Part model, mm, in its own coordinate system. Give positions to 0.01 mm unless a question says otherwise; leave off trailing zeros. Order: outer loops, then holes, each group sorted by start corner. A loop starts at its lowest first (then second) coordinate and runs counter-clockwise, first axis right, second up. Notation, with made-up numbers: (50, -36.5) -> (73, -36.5) arc R10 ccw to (73, -22.5) -> close; hole circle Ø7 at (49.5, 44). An arc over 180 degrees is marked (long way). Write item = value, one per line. Start each with the question number.
Item 1: Drill centre lines: line 1 along Y through (x, z) = (153.5, -387); line 2 along X through (y, z) = (753, 286); line 3 along Z through (x, y) = (-231.5, 44). Where is each one in solid material? Low to high.
Item 2: Flat gauge pins, fed straight in: P1, Ø9, axis at y = 278.5, z = -481.5, coming from the +X side; P2, Ø6, axis at x = -456, z = -478.5, coming from the -Y side; P3, Ø12, axis at y = 41, z = -262, coming from the +X side. Where does each tip first touch, or does it go through?
Item 3: Band-saw the part on D-D on x = -886.5. Write the cut outline in (y, z), plus the area to 3 significant figures.
Item 4: Band-saw the part on C-C on z = 53.5. Write the cut outline in (x, y).
Item 5: Band-saw the part on B-B on y = 676. Write the cut outline in (x, z), plus the area to 3 significant figures.
Item 6: Band-saw the part on A-A on x = 308. Write the cut outline in (y, z).
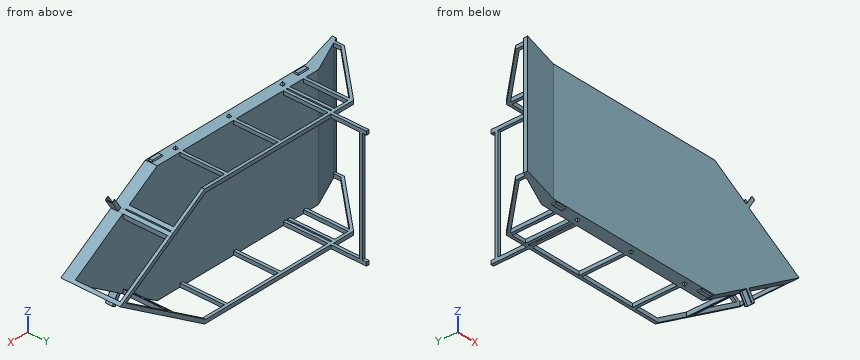
```python
from build123d import *

# Parameters (mm, degrees)
BOSS_EXTRUDE1_DEPTH      = 500
BOSS_EXTRUDE2_DEPTH      = 500
BOSS_EXTRUDE2_DEPTH_BACK = 500
CUT_EXTRUDE1_START       = -500
CUT_EXTRUDE1_OUTLINE_W   = 473.864747831
CUT_EXTRUDE1_OUTLINE_H   = 375
CUT_EXTRUDE1_OUTLINE_W_2 = 7.552750907
CUT_EXTRUDE1_OUTLINE_W_3 = 441.311996924
CUT_EXTRUDE1_OUTLINE_W_4 = 436.609859473
CUT_EXTRUDE1_OUTLINE_W_5 = 473.864747832
CUT_EXTRUDE1_OUTLINE_W_6 = 12.254888358
CUT_EXTRUDE1_OUTLINE_W_7 = 125
CUT_EXTRUDE1_DEPTH       = 1000
BOSS_EXTRUDE3_DEPTH      = 100
CUT_EXTRUDE4_DEPTH       = 470
BOSS_EXTRUDE5_DEPTH      = 500
BOSS_EXTRUDE5_DEPTH_BACK = 500
CUT_EXTRUDE7_DEPTH       = 470
SKETCH10_W               = 1000
SKETCH10_H               = 25
BOSS_EXTRUDE6_DEPTH      = 25
SKETCH11_W               = 25
SKETCH11_H               = 25
SKETCH11_W_2             = 24.921787331
BOSS_EXTRUDE7_DEPTH      = 25
BOSS_EXTRUDE7_TAPER      = 30
BOSS_EXTRUDE8_START      = 525.229495663
BOSS_EXTRUDE8_DEPTH      = 0.022340747
BOSS_EXTRUDE8_START_2    = -485
BOSS_EXTRUDE8_2_DEPTH    = 25
BOSS_EXTRUDE8_START_3    = 13.864747831
BOSS_EXTRUDE8_3_DEPTH    = 25
BOSS_EXTRUDE8_START_4    = 512.729495663
BOSS_EXTRUDE8_4_DEPTH    = 25.022340747
BOSS_EXTRUDE8_START_5    = 37
BOSS_EXTRUDE8_5_DEPTH    = 26
BOSS_EXTRUDE10_DEPTH     = 500
CUT_EXTRUDE8_DEPTH       = 440
CUT_EXTRUDE9_DEPTH       = 23
CUT_EXTRUDE10_DEPTH      = 23
SKETCH20_W               = 100
SKETCH20_H               = 40
BOSS_EXTRUDE11_DEPTH     = 10
BOSS_EXTRUDE11_TAPER     = 29
SKETCH22_W               = 100
SKETCH22_H               = 40
BOSS_EXTRUDE12_DEPTH     = 10
BOSS_EXTRUDE12_TAPER     = 29


with BuildPart() as part:
    # Sketch3 → Boss-Extrude1 (new body)
    with BuildSketch(Plane(origin=(0, 0, 0), x_dir=(1, 0, 0), z_dir=(0, 1, 0))):
        Polygon((750, -500), (1535.458991325, 0), (750, 500), (-750, 500), (-750, -500), align=None)
        Polygon((741.261584038, -470), (1479.593035884, 0), (741.261584038, 470), (-720, 470), (-720, -470), align=None, mode=Mode.SUBTRACT)
    extrude(amount=BOSS_EXTRUDE1_DEPTH)

    # Sketch4 → Boss-Extrude2 (add, two sides: drawn at the far end of the back side and taken through both)
    with BuildSketch(Plane.XY.offset(-BOSS_EXTRUDE2_DEPTH_BACK)):
        Polygon((-750, 0), (-750, 100), (-1044.23243351, -38.029978885), (-1044.23243351, 21.970021115), (-635, 466.05675301), (-635, 500), (-1066.865697626, 31.352330432), (-1066.865697626, -48.647669568), (-1096.782201963, -62.68206548), (-1096.782201963, -97.017235637), align=None)
    extrude(amount=BOSS_EXTRUDE2_DEPTH + BOSS_EXTRUDE2_DEPTH_BACK)

    # Cut-Extrude1: read off the stored shape, not the designer's step
    # Cut-Extrude1 outline → Cut-Extrude1 (cut)
    with BuildSketch(Plane.XY.offset(CUT_EXTRUDE1_START)):
        Polygon((-635, 100), (-635, 466.05675301), (-750, 341.262210872), (-750, 100), align=None)
        with Locations((774.661869579, 287.5)):
            Rectangle(CUT_EXTRUDE1_OUTLINE_W, CUT_EXTRUDE1_OUTLINE_H)
        with Locations((1040.370618948, 287.5)):
            Rectangle(CUT_EXTRUDE1_OUTLINE_W_2, CUT_EXTRUDE1_OUTLINE_H)
        with Locations((1289.802992863, 287.5)):
            Rectangle(CUT_EXTRUDE1_OUTLINE_W_3, CUT_EXTRUDE1_OUTLINE_H)
        with Locations((-204.440181906, 287.5)):
            Rectangle(CUT_EXTRUDE1_OUTLINE_W_4, CUT_EXTRUDE1_OUTLINE_H)
        with Locations((275.797121747, 287.5)):
            Rectangle(CUT_EXTRUDE1_OUTLINE_W_5, CUT_EXTRUDE1_OUTLINE_H)
        with Locations((-453.872555821, 287.5)):
            Rectangle(CUT_EXTRUDE1_OUTLINE_W_6, CUT_EXTRUDE1_OUTLINE_H)
        with Locations((-547.5, 287.5)):
            Rectangle(CUT_EXTRUDE1_OUTLINE_W_7, CUT_EXTRUDE1_OUTLINE_H)
        Polygon((-750, 375.205457862), (-635, 500), (-750, 500), align=None)
    extrude(amount=CUT_EXTRUDE1_DEPTH, mode=Mode.SUBTRACT)

    # Sketch3<6> → Boss-Extrude3 (add)
    with BuildSketch(Plane(origin=(0, 0, 0), x_dir=(1, 0, 0), z_dir=(0, 1, 0))):
        Polygon((750, -500), (1535.458991325, 0), (750, 500), (-750, 500), (-750, -500), align=None)
    extrude(amount=BOSS_EXTRUDE3_DEPTH)

    # Sketch4<6> → Cut-Extrude4 (cut, symmetric)
    with BuildSketch(Plane.XY):
        Polygon((-1066.865697626, -48.647669568), (-1044.23243351, -38.029978885), (-1044.23243351, 21.970021115), (-750, 341.262210872), (-635, 466.05675301), (-635, 500), (-750, 375.205457862), (-1066.865697626, 31.352330432), align=None)
    extrude(amount=CUT_EXTRUDE4_DEPTH, both=True, mode=Mode.SUBTRACT)

    # Sketch4<7> → Boss-Extrude5 (add, two sides: drawn at the far end of the back side and taken through both)
    with BuildSketch(Plane.XY.offset(-BOSS_EXTRUDE5_DEPTH_BACK)):
        Polygon((-447.745111642, 475), (-447.745111642, 100), (-422.745111642, 100), (-422.745111642, 475), (-422.745111642, 500), (-422.745111642, 800), (-447.745111642, 800), (-447.745111642, 500), align=None)
    extrude(amount=BOSS_EXTRUDE5_DEPTH + BOSS_EXTRUDE5_DEPTH_BACK)

    # Sketch4<8> → Cut-Extrude7 (cut, symmetric)
    with BuildSketch(Plane.XY):
        Polygon((-447.745111642, 475), (-447.745111642, 100), (-422.745111642, 100), (-422.745111642, 475), (-422.745111642, 500), (-422.745111642, 800), (-447.745111642, 800), (-447.745111642, 500), align=None)
    extrude(amount=CUT_EXTRUDE7_DEPTH, both=True, mode=Mode.SUBTRACT)

    # Sketch10 → Boss-Extrude6 (add)
    with BuildSketch(Plane.ZY.offset(447.745111642)):
        with Locations((0, 752.218873566)):
            Rectangle(SKETCH10_W, SKETCH10_H)
    extrude(amount=-BOSS_EXTRUDE6_DEPTH)

    # Sketch11 → Boss-Extrude7 (add)
    with BuildSketch(Plane.XY.offset(500)):
        with Locations((525.229495663, 50)):
            Rectangle(SKETCH11_W, SKETCH11_H)
        with Locations((26.364747831, 50)):
            Rectangle(SKETCH11_W, SKETCH11_H)
        with Locations((-472.460893666, 50)):
            Rectangle(SKETCH11_W_2, SKETCH11_H)
    extrude(amount=BOSS_EXTRUDE7_DEPTH, taper=BOSS_EXTRUDE7_TAPER)

    # Boss-Extrude8: read off the stored shape, not the designer's step
    # Boss-Extrude8 outline → Boss-Extrude8 (add)
    with BuildSketch(Plane.YZ.offset(BOSS_EXTRUDE8_START)):
        Polygon((62.5, -500), (37.5, -500), (50, -521.650635095), align=None)
    extrude(amount=BOSS_EXTRUDE8_DEPTH)

    # Boss-Extrude8 2 outline → Boss-Extrude8 2 (add)
    with BuildSketch(Plane.YZ.offset(BOSS_EXTRUDE8_START_2)):
        Polygon((62.5, -500), (37.5, -500), (50, -521.650635095), align=None)
    extrude(amount=BOSS_EXTRUDE8_2_DEPTH)

    # Boss-Extrude8 3 outline → Boss-Extrude8 3 (add)
    with BuildSketch(Plane.YZ.offset(BOSS_EXTRUDE8_START_3)):
        Polygon((62.5, -500), (37.5, -500), (50, -521.650635095), align=None)
    extrude(amount=BOSS_EXTRUDE8_3_DEPTH)

    # Boss-Extrude8 4 outline → Boss-Extrude8 4 (add)
    with BuildSketch(Plane.YZ.offset(BOSS_EXTRUDE8_START_4)):
        Polygon((62.5, -500), (37.5, -500), (50, -521.650635095), align=None)
    extrude(amount=BOSS_EXTRUDE8_4_DEPTH)

    # Boss-Extrude8 5 outline → Boss-Extrude8 5 (cut)
    with BuildSketch(Plane(origin=(0, 0, 0), x_dir=(1, 0, 0), z_dir=(0, 1, 0)).offset(BOSS_EXTRUDE8_START_5)):
        Polygon((512.729495663, 500), (525.229495663, 521.650635095), (525.240666036, 521.669982749), (524.472780219, 523), (512.729495663, 523), align=None)
        Polygon((526.008551854, 523), (525.240666036, 521.669982749), (525.25183641, 521.650635095), (537.75183641, 500), (537.75183641, 523), align=None)
        Polygon((38.864747831, 500), (38.864747831, 523), (13.864747831, 523), (13.864747831, 500), (26.364747831, 521.650635095), align=None)
        Polygon((-460, 500), (-460, 523), (-485, 523), (-485, 500), (-472.5, 521.650635095), align=None)
    extrude(amount=BOSS_EXTRUDE8_5_DEPTH, mode=Mode.SUBTRACT)

    # Sketch15 → Boss-Extrude10 (add)
    with BuildSketch(Plane(origin=(0, 500, 0), x_dir=(1, 0, 0), z_dir=(0, 1, 0))):
        Polygon((1069.146994401, -296.84044748), (1044.146994401, -312.754709253), (1097.846962052, -397.112954104), (1122.846962052, -381.198692331), align=None)
        Polygon((1044.146994401, 312.754709253), (1097.846962052, 397.112954104), (1122.846962052, 381.198692331), (1069.146994401, 296.84044748), align=None)
    extrude(amount=-BOSS_EXTRUDE10_DEPTH)

    # Sketch15<2> → Cut-Extrude8 (cut)
    with BuildSketch(Plane(origin=(0, 500, 0), x_dir=(1, 0, 0), z_dir=(0, 1, 0))):
        Polygon((1069.146994401, -296.84044748), (1044.146994401, -312.754709253), (1097.846962052, -397.112954104), (1122.846962052, -381.198692331), align=None)
        Polygon((1044.146994401, 312.754709253), (1097.846962052, 397.112954104), (1122.846962052, 381.198692331), (1069.146994401, 296.84044748), align=None)
    extrude(amount=-CUT_EXTRUDE8_DEPTH, mode=Mode.SUBTRACT)

    # Sketch17 → Cut-Extrude9 (cut)
    with BuildSketch(Plane(origin=(601.368753994, 0, -382.813590929), x_dir=(0.5369996765096833, 0, 0.8435824485066624), z_dir=(-0.8435824485066624, 0, 0.5369996765096833))):
        Polygon((824.540981636, 5), (919.540981636, 5), (968.552500425, 5), (968.552500425, 55), (924.540981636, 55), (824.540981636, 55), align=None)
    extrude(amount=-CUT_EXTRUDE9_DEPTH, mode=Mode.SUBTRACT)

    # Sketch19 → Cut-Extrude10 (cut)
    with BuildSketch(Plane(origin=(601.368753994, 0, 382.813590929), x_dir=(-0.5369996765096847, 0, 0.8435824485066614), z_dir=(-0.8435824485066615, 0, -0.5369996765096847))):
        Polygon((-829.540981636, 55), (-824.540981636, 55), (-824.540981636, 5), (-829.540981636, 5), (-919.540981636, 5), (-930.414815986, 5), (-930.414815986, 55), (-919.540981636, 55), align=None)
    extrude(amount=-CUT_EXTRUDE10_DEPTH, mode=Mode.SUBTRACT)

    # Sketch20 → Boss-Extrude11 (add)
    with BuildSketch(Plane.XY.offset(500)):
        with Locations((689.590277632, 30.409722368)):
            Rectangle(SKETCH20_W, SKETCH20_H)
    boss_extrude11 = extrude(amount=BOSS_EXTRUDE11_DEPTH, taper=BOSS_EXTRUDE11_TAPER)

    # Mirror1: Boss-Extrude11 across plane
    add(boss_extrude11.mirror(Plane.XY))

    # Sketch22 → Boss-Extrude12 (add)
    with BuildSketch(Plane.XY.offset(500)):
        with Locations((-666.276639524, 30.409722368)):
            Rectangle(SKETCH22_W, SKETCH22_H)
    boss_extrude12 = extrude(amount=BOSS_EXTRUDE12_DEPTH, taper=BOSS_EXTRUDE12_TAPER)

    # Mirror2: Boss-Extrude12 across plane
    add(boss_extrude12.mirror(Plane.XY))


solid = part.part
```
Values found:
q1.line_1 = 0 to 100
q1.line_2 = -447.75 to -422.75
q1.line_3 = -500 to 500
q2.P1 = 537.73
q2.P2 = 0
q2.P3 = 1133.3
q3.outline = (-38.19, -500) -> (35.97, -500) -> (35.97, 500) -> (-38.19, 500) -> close; (193.14, -500) -> (227.08, -500) -> (227.08, -470) -> (193.14, -470) -> close; (193.14, 470) -> (227.08, 470) -> (227.08, 500) -> (193.14, 500) -> close
q3.area = 76,200 mm^2
q4.outline = (-1096.78, -97.02) -> (-750, 0) -> (1451.41, 0) -> (1451.41, 100) -> (-750, 100) -> (-1096.78, -62.68) -> close; (-447.75, 739.72) -> (-422.75, 739.72) -> (-422.75, 764.72) -> (-447.75, 764.72) -> close; (1395.55, 475) -> (1451.41, 475) -> (1451.41, 500) -> (1395.55, 500) -> close
q5.outline = (-447.75, -500) -> (-422.75, -500) -> (-422.75, -470) -> (-447.75, -470) -> close; (-447.75, 470) -> (-422.75, 470) -> (-422.75, 500) -> (-447.75, 500) -> close
q5.area = 1,500 mm^2
q6.outline = (0, -500) -> (100, -500) -> (100, 500) -> (0, 500) -> close; (475, -500) -> (500, -500) -> (500, -470) -> (475, -470) -> close; (475, 470) -> (500, 470) -> (500, 500) -> (475, 500) -> close
